Geometry check sheet. Reference: the model listing, model coordinates, mm. Give positions to 0.01 mm unless a question says otherwise; leave off trailing zeros. Write each loop counter-clockwise with the first axis right and the second up, starting at its lowest first coordinate (ties: lowest second). Pieces come first, ordered by that corner, then holes. Notation, with made-up numbers: M 82,16 L 87,16 A20 cw 87,25 Z; hole C 52,7 d7. An arc over 180 degrees is marked long. One line per item, written item: value. Start each with the question number.
1. Scan lines: line 1 (Z direction, x = 9, y = 2.2); line 2 (Z direction, x = 17.5, y = 0.3); line 3 (X direction, y = 1.8, z = -95). Record each from-to range of solid material in increasing order.
2. Cross-section at B-B on z = -237. Record the cut outline in (x, y), then the cut area to 3 significant figures.
3. Cross-section at C-C on x = 46.5. Record the cut outline in (y, z).
4. Cross-section at A-A on y = 0.7. Count the separate pieces of the cut face and the enclosed holes in it, then the cut area to 3 significant figures.
5. Gauge pin test, flat ends, axial feed: pin 1 (1.5 mm diameter, centred on y = 1.5, z = -17.5, fed in from +X); pin 2 (1 mm diameter, centred on y = 1, z = -65, fed in from -X); pin 3 (1.5 mm diameter, centred on x = -1, y = 1, fed in from +Z); pin 4 (3 mm diameter, centred on x = 77, z = -35.5, fed in from +Y). Record the tip position at first contact, or that the pin passes through.
from build123d import *

# Parameters (mm, degrees)
SALIENTE_EXTRUIR1_DEPTH = 3.2
CORTAR_EXTRUIR1_DEPTH   = 3.2
REDONDEO1_R             = 3
CROQUIS3_R              = 2.05
CORTAR_EXTRUIR2_DEPTH   = 3.2
CORTAR_EXTRUIR3_DEPTH   = 3.2
CROQUIS5_R              = 1.55
CORTAR_EXTRUIR4_DEPTH   = 3.2


with BuildPart() as part:
    # Croquis1 → Saliente-Extruir1 (new body)
    with BuildSketch(Plane(origin=(0, 0, 0), x_dir=(1, 0, 0), z_dir=(0, 1, 0))):
        Polygon((7, 66.1), (10, 66.1), (10, 62.9), (7, 62.9), (7, 61.5), (3, 61.5), (3, 62.9), (0, 62.9), (0, 57), (-3, 57), (-3, 51), (0, 51), (0, 0), (165, 0), (165, 1.5), (168, 1.5), (168, 7.5), (165, 7.5), (165, 13.4), (162, 13.4), (162, 12), (158, 12), (158, 13.4), (155, 13.4), (155, 16.6), (158, 16.6), (158, 18), (162, 18), (162, 16.6), (165, 16.6), (165, 22.5), (168, 22.5), (168, 28.5), (165, 28.5), (165, 377), (30, 377), (30, 373.9), (21.6, 373.9), (21.6, 370.9), (23, 370.9), (23, 366.9), (21.6, 366.9), (21.6, 363.9), (18.4, 363.9), (18.4, 366.9), (17, 366.9), (17, 370.9), (18.4, 370.9), (18.4, 373.9), (10, 373.9), (10, 377), (0, 377), (0, 358), (-3, 358), (-3, 352), (0, 352), (0, 346.1), (3, 346.1), (3, 347.5), (7, 347.5), (7, 346.1), (10, 346.1), (10, 342.9), (7, 342.9), (7, 341.5), (3, 341.5), (3, 342.9), (0, 342.9), (0, 337), (-3, 337), (-3, 331), (0, 331), (0, 218), (-3, 218), (-3, 212), (0, 212), (0, 206.1), (3, 206.1), (3, 207.5), (7, 207.5), (7, 206.1), (10, 206.1), (10, 202.9), (7, 202.9), (7, 201.5), (3, 201.5), (3, 202.9), (0, 202.9), (0, 197), (-3, 197), (-3, 191), (0, 191), (0, 78), (-3, 78), (-3, 72), (0, 72), (0, 66.1), (3, 66.1), (3, 67.5), (7, 67.5), align=None)
    extrude(amount=SALIENTE_EXTRUIR1_DEPTH)

    # Croquis2 → Cortar-Extruir1 (cut)
    with BuildSketch(Plane.XZ):
        with BuildLine():
            Line((165, -377), (33, -377))
            ThreePointArc((33, -377), (68.343071274, -192.304293087), (165, -31))
            Line((165, -31), (165, -377))
        make_face()
    extrude(amount=-CORTAR_EXTRUIR1_DEPTH, mode=Mode.SUBTRACT)

    # Redondeo1
    redondeo1_edges = [part.edges().sort_by_distance(p)[0] for p in [
        (33, 1.6, -377),
    ]]
    fillet(redondeo1_edges, radius=REDONDEO1_R)

    # Croquis3 → Cortar-Extruir2 (cut)
    with BuildSketch(Plane(origin=(0, 3.2, 0), x_dir=(1, 0, 0), z_dir=(0, 1, 0))):
        with Locations(Location((40, 80, 0), (0, 0, 270))):
            Circle(CROQUIS3_R)
        with Locations(Location((90, 80, 0), (0, 0, 270))):
            Circle(CROQUIS3_R)
        with Locations(Location((40, 230, 0), (0, 0, 270))):
            Circle(CROQUIS3_R)
    extrude(amount=-CORTAR_EXTRUIR2_DEPTH, mode=Mode.SUBTRACT)

    # Croquis4 → Cortar-Extruir3 (cut)
    with BuildSketch(Plane.XZ):
        with BuildLine():
            Line((143, -30.5), (129, -30.5))
            ThreePointArc((129, -30.5), (127.585786438, -31.085786438), (127, -32.5))
            Line((127, -32.5), (127, -38.5))
            ThreePointArc((127, -38.5), (127.585786438, -39.914213562), (129, -40.5))
            Line((129, -40.5), (143, -40.5))
            ThreePointArc((143, -40.5), (144.414213562, -39.914213562), (145, -38.5))
            Line((145, -38.5), (145, -32.5))
            ThreePointArc((145, -32.5), (144.414213562, -31.085786438), (143, -30.5))
        make_face()
    extrude(amount=-CORTAR_EXTRUIR3_DEPTH, mode=Mode.SUBTRACT)

    # Croquis5 → Cortar-Extruir4 (cut)
    with BuildSketch(Plane.XZ):
        with Locations(Location((110, -95, 0), (0, 0, 270))):
            Circle(CROQUIS5_R)
        with Locations(Location((35, -95, 0), (0, 0, 270))):
            Circle(CROQUIS5_R)
        with Locations(Location((15, -175, 0), (0, 0, 270))):
            Circle(CROQUIS5_R)
        with Locations(Location((60, -175, 0), (0, 0, 270))):
            Circle(CROQUIS5_R)
        with Locations(Location((77, -35.5, 0), (0, 0, 270))):
            Circle(CROQUIS5_R)
        with Locations(Location((37, -215.5, 0), (0, 0, 270))):
            Circle(CROQUIS5_R)
        with Locations(Location((57, -155.5, 0), (0, 0, 270))):
            Circle(CROQUIS5_R)
    extrude(amount=-CORTAR_EXTRUIR4_DEPTH, mode=Mode.SUBTRACT)


solid = part.part
Report:
1. line 1: z = -377 to -346.1, -342.9 to -206.1, -202.9 to -66.1, -62.9 to 0
1. line 2: z = -373.9 to -370.9, -366.9 to 0
1. line 3: x = 0 to 33.45, 36.55 to 108.45, 111.55 to 117.24
2. outline: M 0,0 L 53.49,0 L 53.49,3.2 L 0,3.2 Z
2. area: 171 mm^2
3. outline: M 0,-264.29 L 3.2,-264.29 L 3.2,0 L 0,0 Z
4. separate pieces: 1
4. enclosed holes: 11
4. area: 30,800 mm^2
5. pin 1: stops at x = 165
5. pin 2: stops at x = 10
5. pin 3: stops at z = -51
5. pin 4: passes through
